```python
from build123d import *

# Parameters (mm, degrees)
SKETCH_1_W             = 35
SKETCH_1_H             = 42
EXTRUDE_1_DEPTH        = 4
SKETCH_4_R             = 10
EXTRUDE_2_DEPTH        = 3.5
CUT_EXTRUDE_START      = -2
CUT_EXTRUDE_2_DEPTH    = 2
SKETCH_6_R             = 2.6
CUT_EXTRUDE_3_DEPTH    = 30.656365253
SKETCH_7_R             = 5
CUT_EXTRUDE_4_DEPTH    = 5
CHAMFER_1_SIZE         = 0.5
CHAMFER_2_SIZE         = 0.5
CHAMFER_3_SIZE         = 1
CUT_EXTRUDE_5_DEPTH    = 30.656365253
FILLET_1_R             = 3
HOLE_WIZARD_M4_1_D     = 3.3
HOLE_WIZARD_M4_1_DEPTH = 8
SKETCH_14_W            = 15
SKETCH_14_H            = 5
CUT_EXTRUDE_6_DEPTH    = 29.482450737
FILLET_2_R             = 2
FILLET_3_R             = 2


with BuildPart() as part:
    # 草图1 → 凸台-拉伸1 (new, symmetric)
    with BuildSketch(Plane.XY):
        Rectangle(SKETCH_1_W, SKETCH_1_H)
    extrude(amount=EXTRUDE_1_DEPTH, both=True)

    # 草图4 → 凸台-拉伸2 (add)
    with BuildSketch(Plane(origin=(0, 0, -4), x_dir=(-1, 0, 0), z_dir=(0, 0, -1))):
        with Locations(Location((0, 0, 0), (0, 0, 180))):
            Circle(SKETCH_4_R)
        with BuildLine():
            Line((-5, 6), (5, 6))
            ThreePointArc((5, 6), (5.707106781, 5.707106781), (6, 5))
            Line((6, 5), (6, -5))
            ThreePointArc((6, -5), (5.707106781, -5.707106781), (5, -6))
            Line((5, -6), (-5, -6))
            ThreePointArc((-5, -6), (-5.707106781, -5.707106781), (-6, -5))
            Line((-6, -5), (-6, 5))
            ThreePointArc((-6, 5), (-5.707106781, 5.707106781), (-5, 6))
        make_face(mode=Mode.SUBTRACT)
    extrude(amount=EXTRUDE_2_DEPTH)

    # 草图5 → 切除-拉伸2 (cut)
    with BuildSketch(Plane(origin=(0, 0, -4), x_dir=(-1, 0, 0), z_dir=(0, 0, -1)).offset(CUT_EXTRUDE_START)):
        with BuildLine():
            Line((6, -5), (6, 5))
            ThreePointArc((6, 5), (5.707106781, 5.707106781), (5, 6))
            Line((5, 6), (-5, 6))
            ThreePointArc((-5, 6), (-5.707106781, 5.707106781), (-6, 5))
            Line((-6, 5), (-6, -5))
            ThreePointArc((-6, -5), (-5.707106781, -5.707106781), (-5, -6))
            Line((-5, -6), (5, -6))
            ThreePointArc((5, -6), (5.707106781, -5.707106781), (6, -5))
        make_face()
    extrude(amount=CUT_EXTRUDE_2_DEPTH, mode=Mode.SUBTRACT)

    # 草图6 → 切除-拉伸3 (cut, through all)
    with BuildSketch(Plane.XY.offset(4)):
        Circle(SKETCH_6_R)
    extrude(amount=-CUT_EXTRUDE_3_DEPTH, mode=Mode.SUBTRACT)

    # 草图7 → 切除-拉伸4 (cut)
    with BuildSketch(Plane.XY.offset(4)):
        Circle(SKETCH_7_R)
    extrude(amount=-CUT_EXTRUDE_4_DEPTH, mode=Mode.SUBTRACT)

    # 倒角1
    chamfer_1_edges = [part.edges().sort_by_distance(p)[0] for p in [
        (-5.707106781, 5.707106781, -7.5),
        (0, 6, -7.5),
        (5.707106781, 5.707106781, -7.5),
        (6, 0, -7.5),
        (5.707106781, -5.707106781, -7.5),
        (0, -6, -7.5),
        (-5.707106781, -5.707106781, -7.5),
        (-6, 0, -7.5),
    ]]
    chamfer(chamfer_1_edges, length=CHAMFER_1_SIZE)

    # 倒角2
    chamfer_2_edges = [part.edges().sort_by_distance(p)[0] for p in [
        (-5, 0, 4),
    ]]
    chamfer(chamfer_2_edges, length=CHAMFER_2_SIZE)

    # 倒角3
    chamfer_3_edges = [part.edges().sort_by_distance(p)[0] for p in [
        (-10, 0, -4),
    ]]
    chamfer(chamfer_3_edges, length=CHAMFER_3_SIZE)

    # 草图10 → 切除-拉伸5 (cut, through all)
    with BuildSketch(Plane.XY.offset(4)):
        Polygon((11, -13), (17.5, -13), (17.5, 13), (11, 13), (11, 0), align=None)
        with BuildLine():
            ThreePointArc((8.8, 6.6), (10.435516279, 3.478505426), (11, 0))
            Line((11, 0), (11, 13))
            Line((11, 13), (4, 13))
            Line((4, 13), (8.8, 6.6))
        make_face()
        with BuildLine():
            Line((4, -13), (11, -13))
            Line((11, -13), (11, 0))
            ThreePointArc((11, 0), (10.435516279, -3.478505426), (8.8, -6.6))
            Line((8.8, -6.6), (4, -13))
        make_face()
    cut_extrude_5 = extrude(amount=-CUT_EXTRUDE_5_DEPTH, mode=Mode.SUBTRACT)

    # 镜向1: 切除-拉伸5 across plane
    add(cut_extrude_5.mirror(Plane(origin=(0, 0, 0), x_dir=(0, 0, 1), z_dir=(1, 0, 0))), mode=Mode.SUBTRACT)

    # 圆角1
    fillet_1_edges = [part.edges().sort_by_distance(p)[0] for p in [
        (4, 13, 0),
        (4, -13, 0),
        (-4, -13, 0),
        (-4, 13, 0),
    ]]
    fillet(fillet_1_edges, radius=FILLET_1_R)

    # M4 螺纹孔1
    with Locations(Plane(origin=(0, 21, 0), x_dir=(1, 0, 0), z_dir=(0, 1, 0))):
        with Locations((12.5, 0), (-12.5, 0)):
            hole_wizard_m4_1 = Hole(HOLE_WIZARD_M4_1_D / 2, depth=HOLE_WIZARD_M4_1_DEPTH)

    # 镜向2: M4 螺纹孔1 across plane
    add(hole_wizard_m4_1.mirror(Plane.ZX), mode=Mode.SUBTRACT)

    # 草图14 → 切除-拉伸6 (cut, through all)
    with BuildSketch(Plane(origin=(0, 0, -4), x_dir=(-1, 0, 0), z_dir=(0, 0, -1))):
        with Locations((0, 18.5)):
            Rectangle(SKETCH_14_W, SKETCH_14_H)
        with Locations((0, -18.5)):
            Rectangle(SKETCH_14_W, SKETCH_14_H)
    extrude(amount=-CUT_EXTRUDE_6_DEPTH, mode=Mode.SUBTRACT)

    # 圆角2
    fillet_2_edges = [part.edges().sort_by_distance(p)[0] for p in [
        (17.5, 13, 0),
        (17.5, -13, 0),
        (-17.5, 13, 0),
        (-17.5, -13, 0),
        (17.5, -21, 0),
        (-17.5, -21, 0),
        (-17.5, 21, 0),
        (17.5, 21, 0),
    ]]
    fillet(fillet_2_edges, radius=FILLET_2_R)

    # 圆角3
    fillet_3_edges = [part.edges().sort_by_distance(p)[0] for p in [
        (7.5, 16, 0),
        (7.5, 21, 0),
        (-7.5, 21, 0),
        (-7.5, 16, 0),
        (7.5, -16, 0),
        (-7.5, -16, 0),
        (-7.5, -21, 0),
        (7.5, -21, 0),
    ]]
    fillet(fillet_3_edges, radius=FILLET_3_R)


solid = part.part
```
The listing builds one solid part. Answer for the finished solid, in the listing's coordinates (mm). A direction names the side the tool comes from. Coordinates: 2 decimals unless noted, no trailing zeros. Write each loop counter-clockwise with the first axis right and the second up, starting at its lowest first coordinate (ties: lowest second). Pieces come first, ordered by that corner, then holes. Notation, with made-up numbers: (55.25, 78) - (89.25, 78) arc R17 cw to (89.25, 84) - close; hole circle Ø7 at (66.25, 35.5). An arc over 180 degrees is marked (long way). Return JSON: item names as keys, results as strings. Group by question number.
1. A cutting plane is placed at A-A, the plane y = 18.5. Determine the outline of the cut face in (x, z), plus the area to 3 significant figures.
2. Determine the mould class of faces 1 (the cylindrical face through (-14.024, 16.944, 0.632)), 2 (the flat face through (0, -6, -4)), 3 (the cylindrical face through (-16.9, -20.43, 0.06)) for opening direction Y: released by +Y, released by -Y, zero draft, split by the parting line, or undercut.
3. Given pin 1 (5 mm diameter, centred on x = 0, y = 0, fed in from +Z) (1 decimal); pin 2 (6 mm diameter, centred on x = -3.5, z = -2, fed in from +Y); pin 3 (1.5 mm diameter, centred on x = 5, z = -5, fed in from +Y); pin 4 (6 mm diameter, centred on y = 4, z = 2.5, fed in from -X), each flat-ended and moving along its own axis, determine where each tip first touches the part or whether it passes through.
4. A cutting plane is placed at D-D, the plane z = -6. Determine the outline of the cut face in (x, y), plus the area to 3 significant figures.
5. Which of the six approach directions +Z, -Z, +X, -X, +Y, -Y give full straight-line access (tool end or side, diameter ignored) to faces 4 (the cylindrical face through (-5.715, -5.699, -4.465)), 5 (the cylindrical face through (8.07, 20.4, 0.06)), 6 (the flat face through (0, -16, 0)), 7 (the cylindrical face through (-16.9, 13.57, -0.06)), 8 (the cylindrical face through (16.9, -13.57, -0.06))?
6. Straight lines are drawn through the part: L1, parallel to X at y = -19, z = 2.75; L2, parallel to Y at x = 0, z = -0.25; L3, parallel to Y at x = 14.5, z = 3.25. For each, find the intervals that lie inside material, in ascending order.
7. A cutting plane is placed at C-C, the plane x = 0. Determine the outline of the cut face in (y, z), plus the area to 3 significant figures.
8. A cutting plane is placed at B-B, the plane x = -12.5. Determine the outline of the cut face in (y, z).
Ans:
{
 "1": {"outline": "(-17.5, -4) - (-7.5, -4) - (-7.5, 4) - (-17.5, 4) - close; (7.5, -4) - (17.5, -4) - (17.5, 4) - (7.5, 4) - close; hole circle Ø3.3 at (-12.5, 0); hole circle Ø3.3 at (12.5, 0)", "area": "143 mm²"},
 "2": {"face 1": "zero draft", "face 2": "undercut", "face 3": "released by -Y"},
 "3": {"pin 1": "through", "pin 2": "y = 16.27", "pin 3": "y = 9.6", "pin 4": "x = -10.95"},
 "4": {"outline": "circle Ø20 at (0, 0); hole (-6, -5) arc R1 ccw to (-5, -6) - (5, -6) arc R1 ccw to (6, -5) - (6, 5) arc R1 ccw to (5, 6) - (-5, 6) arc R1 ccw to (-6, 5) - close", "area": "171 mm²"},
 "5": {"face 4": "-Z", "face 5": "+Z, -Z, +Y", "face 6": "+Z, -Z, -Y", "face 7": "+Z, -Z, -X", "face 8": "+Z, -Z, +X"},
 "6": {"L1": "-17.5 to -7.5, 7.5 to 17.5", "L2": "-16 to -5, 5 to 16", "L3": "-21 to -13, 13 to 21"},
 "7": {"outline": "(-16, -4) - (-11, -4) - (-10, -5) - (-10, -7.5) - (-6.5, -7.5) - (-6, -7) - (-6, -2) - (-2.6, -2) - (-2.6, -1) - (-5, -1) - (-5, 3.5) - (-5.5, 4) - (-16, 4) - close; (2.6, -2) - (6, -2) - (6, -7) - (6.5, -7.5) - (10, -7.5) - (10, -5) - (11, -4) - (16, -4) - (16, 4) - (5.5, 4) - (5, 3.5) - (5, -1) - (2.6, -1) - close", "area": "205 mm²"},
 "8": {"outline": "(-21, -4) - (-13, -4) - (-13, -1.65) - (-21, -1.65) - close; (-21, 1.65) - (-13, 1.65) - (-13, 4) - (-21, 4) - close; (13, -4) - (21, -4) - (21, -1.65) - (13, -1.65) - close; (13, 1.65) - (21, 1.65) - (21, 4) - (13, 4) - close"}
}
